Read the model definition and answer for the solid it produces. Units are mm, in the model's axes. A direction names the side the tool comes from. Coordinates: 2 decimals unless noted, no trailing zeros. Order: outer loops, then holes, each group sorted by start corner. A loop starts at its lowest first (then second) coordinate and runs counter-clockwise, first axis right, second up. Notation, with made-up numbers: (-35.5, -6.75) - (17.5, -6.75) arc R19 cw to (17.5, 30.25) - close; hole circle Ø4 at (12.25, 87). An arc over 180 degrees is marked (long way). Write item = value, one per line.
from build123d import *

# Parameters (mm, degrees)
F1_DEPTH = 152.4
F2_W     = 63.5
F2_H     = 12.7
F3_DEPTH = 101.601
F2_W_2   = 55.88
F2_H_2   = 58.42
F4_DEPTH = 25.4
F6_DEPTH = 101.601
F7_R     = 6.35
F8_DEPTH = 63.501


with BuildPart() as f1:
    # F0 (on Right) → F1 (new body)
    with BuildSketch(Plane.YZ):
        Polygon((-17.78, 31.75), (-50.8, 31.75), (-50.8, -31.75), (50.8, -31.75), (50.8, 31.75), (13.97, 31.75), (13.97, 22.86), (-17.78, 22.86), align=None)
    extrude(amount=F1_DEPTH)

    # F2 (on face) → F3 (cut, through all)
    with BuildSketch(Plane.XZ.offset(50.8)):
        with Locations((31.75, -25.4)):
            Rectangle(F2_W, F2_H)
    extrude(amount=-F3_DEPTH, mode=Mode.SUBTRACT)

    # F2 (on face) → F4 (cut)
    with BuildSketch(Plane.XZ.offset(50.8)):
        with Locations((124.46, -2.54)):
            Rectangle(F2_W_2, F2_H_2)
    extrude(amount=-F4_DEPTH, mode=Mode.SUBTRACT)

    # F5 (on face) → F6 (cut, through all)
    with BuildSketch(Plane.XZ.offset(50.8)):
        Polygon((152.4, 26.67), (152.4, 31.75), (76.2, 31.75), (152.4, -31.75), align=None)
    extrude(amount=-F6_DEPTH, mode=Mode.SUBTRACT)

    # F7 (on face) → F8 (cut, through all)
    with BuildSketch(Plane(origin=(0, 0, -31.75), x_dir=(1, 0, 0), z_dir=(0, 0, -1))):
        with BuildLine():
            ThreePointArc((100.425931, 15.782081), (100.093425, 4.725474), (109.728, 10.16))
            ThreePointArc((109.728, 10.16), (108.812526, 13.444575), (106.330069, 15.782081))
            Line((106.330069, 15.782081), (100.425931, 15.782081))
        make_face()
        with BuildLine():
            ThreePointArc((138.842069, 15.782081), (135.89, 16.51), (132.937931, 15.782081))
            Line((132.937931, 15.782081), (138.842069, 15.782081))
        make_face()
        with BuildLine():
            Line((138.842069, 15.782081), (132.937931, 15.782081))
            ThreePointArc((132.937931, 15.782081), (132.605425, 4.725474), (142.24, 10.16))
            ThreePointArc((142.24, 10.16), (141.324526, 13.444575), (138.842069, 15.782081))
        make_face()
        with BuildLine():
            Line((100.425931, 15.782081), (106.330069, 15.782081))
            ThreePointArc((106.330069, 15.782081), (103.378, 16.51), (100.425931, 15.782081))
        make_face()
        with Locations((135.89, -35.56)):
            Circle(F7_R)
        with Locations((103.378, -35.56)):
            Circle(F7_R)
    extrude(amount=-F8_DEPTH, mode=Mode.SUBTRACT)


solid = f1.part
1) The part is cut by section C-C (y = -29). Determine the outline of the cut face in (x, z), and give its area (3 significant figures).
Returned:
outline = (0, -19.05) - (63.5, -19.05) - (63.5, -31.75) - (96.52, -31.75) - (96.52, 14.82) - (76.2, 31.75) - (0, 31.75) - close
area = 5,150 mm^2
2) Determine the mould class of faces 1 (the face through (48, -50.8, 8)), 2 (the face through (38, -34, 31.75)), 3 (the face through (43, -2, 22.86)), 4 (the face through (58, 50.8, 0)) for opening direction Y: pulls with the +Y half, pulls with the -Y half, needs draft (parallel to the pull), parting line crosses it, or undercut.
Returned:
face_1 = pulls with the -Y half
face_2 = needs draft
face_3 = undercut
face_4 = pulls with the +Y half
3) For faces 5 (the face through (112, -25.4, -18)), 6 (the face through (113.77, 10.58, 0.44)), 7 (the face through (43, 13.97, 27)), 8 (the face through (0, -1, 7)), 9 (the face through (63.5, -1, -25)), determine the directions among +Z, -Z, +X, -X, +Y, -Y from which every point of the face is accessible in a straight line to the end or side of a thin tool.
Returned:
face_5 = +Z, -Z, +X, -Y
face_6 = +Z, +X, +Y, -Y
face_7 = +Z, +X, -X
face_8 = +Z, -Z, -X, +Y, -Y
face_9 = -Z, -X, +Y, -Y
4) The part is cut by section B-B (x = 31.5). Determine the outline of the cut face in (y, z).
Returned:
outline = (-50.8, -19.05) - (50.8, -19.05) - (50.8, 31.75) - (13.97, 31.75) - (13.97, 22.86) - (-17.78, 22.86) - (-17.78, 31.75) - (-50.8, 31.75) - close
5) Flat-ended cylindrical pins translate along their axes: pin 1 Ø5 at (x, y) = (32, -2) entering from +Z; pin 2 Ø8 at (x, z) = (109.5, -12.5) entering from -Y; pin 3 Ø14 at (y, z) = (10, -26.5) entering from -X; pin 4 Ø11.5 at (x, y) = (135.89, -10.16) entering from +Z. Find the tip coordinate at first contact, or state that the pin passes through.
Returned:
pin_1 = 22.86
pin_2 = -25.4
pin_3 = 63.5
pin_4 = through
6) The part is cut by section D-D (x = 135.89). Determine the outline of the cut face in (y, z).
Returned:
outline = (-25.4, -31.75) - (-16.51, -31.75) - (-16.51, -17.99) - (-25.4, -17.99) - close; (-3.81, -31.75) - (29.21, -31.75) - (29.21, -17.99) - (-3.81, -17.99) - close; (41.91, -31.75) - (50.8, -31.75) - (50.8, -17.99) - (41.91, -17.99) - close
7) Straight lines are drawn through the part: line 1 along Y through (x, z) = (135.89, -23.75); line 2 along X through (y, z) = (35.56, -20); line 3 along X through (y, z) = (35, -16). For each, find the intervals that lie inside material, in ascending order. Write a range as from..to.
Returned:
line_1 = -25.4..-16.51, -3.81..29.21, 41.91..50.8
line_2 = 63.5..97.03, 109.73..129.54
line_3 = 0..97.05, 109.7..129.56
8) The part is cut by section A-A (y = 35.56). Determine the outline of the cut face in (x, z), and give its area (3 significant figures).
Returned:
outline = (0, -19.05) - (63.5, -19.05) - (63.5, -31.75) - (97.03, -31.75) - (97.03, 14.39) - (76.2, 31.75) - (0, 31.75) - close; (109.73, -31.75) - (129.54, -31.75) - (129.54, -12.7) - (109.73, 3.81) - close; (142.24, -31.75) - (152.4, -31.75) - (142.24, -23.28) - close
area = 5,760 mm^2
